Autodesk Inventor part; units mm, degrees
ref_plane "YZ Plane" through (0, 0, 0) normal (1, 0, 0) x (0, 1, 0)
ref_plane "XZ Plane" through (0, 0, 0) normal (0, 1, 0) x (-1, 0, 0)
ref_plane "XY Plane" through (0, 0, 0) normal (0, 0, 1) x (1, 0, 0)
sketch "Sketch1" plane through (0, 0, 0) normal (0, 0, 1) x (1, 0, 0)
  line L0 (-130, 607) -> (-130, 0)
  line L1 (-130, 0) -> (130, 0)
  line L2 (130, 0) -> (130, 607)
  line L3 (125, 5) -> (125, 602.1317)
  line L4 (-125, 5) -> (-125, 602.1317)
  line L5 (-125, 5) -> (125, 5)
  arc A0 (-153.9793, 646.614) -> (153.9793, 646.614) centre (0, 735.514) ccw
  arc A1 (130, 607) -> (158.3094, 644.114) centre (0, 735.514) ccw
  arc A2 (-158.3094, 644.114) -> (-130, 607) centre (0, 735.514) ccw
  arc A3 (-125, 602.1317) -> (125, 602.1317) centre (0, 735.514) ccw
  line L6 (-158.3094, 644.114) -> (-153.9793, 646.614)
  line L7 (153.9793, 646.614) -> (158.3094, 644.114)
  point P0 (0, 0)
  point P1 (0, 0)
  point P2 (0, 5)
  dimension "d0" = 260
  dimension "d2" = 607
  dimension "d3" = 607
  dimension "d6" = 5
  dimension "d7" = 5
  dimension "d8" = 5
  dimension "d57" = 355.6
  dimension "d61" = 5
  dimension "d64" = 182.8
  dimension "d79" = 130
  dimension "d80" = 120
  dimension "d81" = 158.3094
  dimension "d82" = 153.9793
  dimension "d83" = 153.9793
extrude "Extrusion1" add sketch "Sketch1" along normal mid plane 100
sketch "Sketch5" plane through (0, 0, 0) normal (0, 0, 1) x (1, 0, 0)
  line L0 (-125, 602.1317) -> (-125, 5)
  line L1 (-125, 602.1317) -> (-125, 5)
  line L2 (-125, 5) -> (125, 5)
  line L3 (-125, 5) -> (125, 5)
  line L4 (125, 5) -> (125, 602.1317)
  line L5 (125, 5) -> (125, 602.1317)
  arc A0 (-125, 602.1317) -> (125, 602.1317) centre (0, 735.514) ccw
  point P0 (0, 0)
  point P1 (0, 5)
  dimension "d67" = 365.6
extrude "Extrusion2" add sketch "Sketch5" along normal mid plane 10
sketch "Sketch6" plane through (-130, 0, 50) normal (0, -1, 0) x (1, 0, 0)
  line L0 (5, -100) -> (255, -100)
  line L1 (130, -100) -> (130, 0)
  line L2 (0, 0) -> (260, 0)
  circle A0 centre (180, -77.5) radius 10
  circle A1 centre (180, -22.5) radius 10
  circle A2 centre (80, -77.5) radius 10
  circle A3 centre (80, -22.5) radius 10
  point P0 (130, -50)
  dimension "d72" = 20
  dimension "d73" = 100
  dimension "d74" = 20
  dimension "d75" = 55
  dimension "d76" = 100
  dimension "d84" = 22.5
extrude "Extrusion5" cut sketch "Sketch6" against normal blind 10
properties part number "Fix Saddle Pervecto" material "Steel ASTM A36"
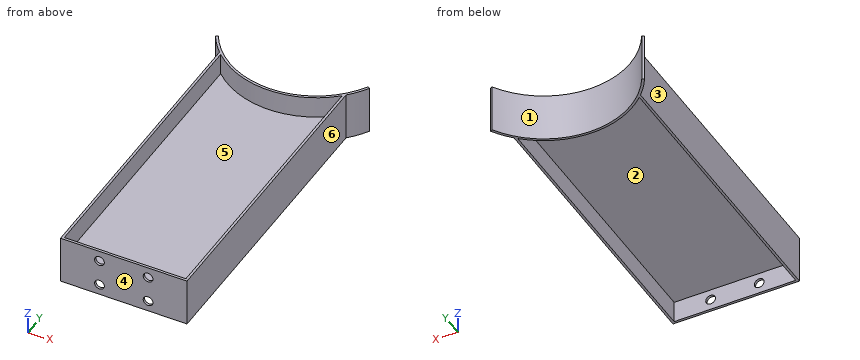
Design review of the part built by this model. Coordinates are the model's own, in mm. Face numbers are marked on the shaded views. A direction names the side the tool comes from. Give positions to 0.01 mm unless a question says otherwise; leave off trailing zeros. Loops run counter-clockwise (first coordinate to the right, second up) from the corner with the lowest first, then second, coordinate; pieces in that order, holes last. Notation, with made-up numbers: (72, 44) -> (88, 44) arc R15 ccw to (88, 56) -> close; hole circle Ø8 at (-16, -9.75). An arc over 180 degrees is marked (long way). One line per item, written item: value.
Q1. We need section D-D on x = -107. Give the boundary of the cut face in (y, z).
Numbers:
outline: (0, -50) -> (5, -50) -> (5, -5) -> (587.3, -5) -> (587.3, -50) -> (593.51, -50) -> (593.51, 50) -> (587.3, 50) -> (587.3, 5) -> (5, 5) -> (5, 50) -> (0, 50) -> close
Q2. Draft analysis for pull direction Y (two halves, no side actions). For the marked faces 4, 5 and 6, state which applies: pulls with the +Y half, pulls with the -Y half, needs draft (parallel to the pull), parting line crosses it, or undercut.
Numbers:
face 4: pulls with the -Y half
face 5: undercut
face 6: needs draft
Q3. Machinability: for the marked faces 1, 2 and 3, which of the approach directions +Z, -Z, +X, -X, +Y, -Y give a long, thin tool a straight path to every point of the face, cutting with its end or side? Answer none if there is none.
Numbers:
face 1: +Z, -Z, +Y
face 2: -Z
face 3: +Z, -Z, -X, -Y
Q4. For L1, parallel to X at y = 3, z = 27; L2, parallel to Z at x = -50, y = 2.5; L3, parallel to X at y = 398, z = -28, list the stretches that pass through material, from the lowest coordinate up.
Numbers:
L1: x = -130 to -59.99, -40.01 to 40.01, 59.99 to 130
L2: z = -50 to -37.5, -17.5 to 17.5, 37.5 to 50
L3: x = -130 to -125, 125 to 130
Q5. We need section A-A on z = 27.5. Give the boundary of the cut face in (x, y).
Numbers:
outline: (-158.31, 644.11) arc R182.8 ccw to (-130, 607) -> (-130, 0) -> (-60, 0) -> (-60, 5) -> (-125, 5) -> (-125, 602.13) arc R182.8 ccw to (125, 602.13) -> (125, 5) -> (60, 5) -> (60, 0) -> (130, 0) -> (130, 607) arc R182.8 ccw to (158.31, 644.11) -> (153.98, 646.61) arc R177.8 cw to (-153.98, 646.61) -> close; (-40, 0) -> (40, 0) -> (40, 5) -> (-40, 5) -> close
Q6. We need section B-B on y = 163.5. Give the boundary of the cut face in (x, z), and give its area (3 significant figures).
Numbers:
outline: (-130, -50) -> (-125, -50) -> (-125, -5) -> (125, -5) -> (125, -50) -> (130, -50) -> (130, 50) -> (125, 50) -> (125, 5) -> (-125, 5) -> (-125, 50) -> (-130, 50) -> close
area: 3,500 mm^2
Q7. We need section C-C on x = 50. Give the boundary of the cut face in (y, z) (3 decimals).
Numbers:
outline: (0, -50) -> (5, -50) -> (5, -37.5) -> (0, -37.5) -> close; (0, -17.5) -> (5, -17.5) -> (5, -5) -> (559.685, -5) -> (559.685, -50) -> (564.889, -50) -> (564.889, 50) -> (559.685, 50) -> (559.685, 5) -> (5, 5) -> (5, 17.5) -> (0, 17.5) -> close; (0, 37.5) -> (5, 37.5) -> (5, 50) -> (0, 50) -> close
Q8. For pin 1 Ø1.5 at (x, z) = (-30.5, 17.5) entering from +Y; pin 2 Ø1 at (x, y) = (-28, 120) entering from -Z; pin 3 Ø8 at (x, z) = (16, 17) entering from +Y; pin 4 Ø2 at (x, z) = (-117.5, -35) entering from -Y, all flat-tipped, find the tip position at first contact; note any pin that passes through.
Numbers:
pin 1: stops at y = 560.48
pin 2: stops at z = -5
pin 3: stops at y = 558.84
pin 4: stops at y = 0
